Input: part model. Units: mm. Frame: model coordinates. A direction names the side the tool comes from. Give positions to 0.01 mm unless a question says otherwise; leave off trailing zeros. Write each loop counter-clockwise with the first axis right and the second up, starting at its lowest first coordinate (ties: lowest second). Pieces come first, ordered by that corner, then holes.
```python
from build123d import *

# Parameters (mm, degrees)
F0_W      = 127
F0_H      = 304.8
F0_W_2    = 76.2
F0_H_2    = 182.88
F1_DEPTH  = 19.05
F2_W      = 101.6
F2_H      = 25.4
F3_DEPTH  = 41.91
F4_W      = 101.6
F4_H      = 208.28
F5_DEPTH  = 12.7
F6_W      = 114.3
F6_H      = 35.56
F7_DEPTH  = 12.7
F8_W      = 85.55
F8_H      = 192.23
F8_W_2    = 79.2
F8_H_2    = 185.88
F8_W_3    = 88.9
F8_H_3    = 3.175
F9_DEPTH  = 3.175
F10_W     = 85.55
F10_H     = 192.23
F10_W_2   = 79.2
F10_H_2   = 185.88
F10_W_3   = 88.9
F10_H_3   = 3.175
F11_DEPTH = 3.175
F13_D     = 15.24
F14_R     = 6.35
F15_W     = 6.35
F15_H     = 242.316
F16_DEPTH = 12.7
F18_DEPTH = 25.4
F19_R     = 3.175
F20_DEPTH = 12.7
F21_R     = 3.175
F22_DEPTH = 12.7


with BuildPart() as f1:
    # F0 (on Front) → F1 (new body, symmetric)
    with BuildSketch(Plane.XZ):
        Rectangle(F0_W, F0_H)
        Rectangle(F0_W_2, F0_H_2, mode=Mode.SUBTRACT)
    extrude(amount=F1_DEPTH, both=True)

    # F2 (on face) → F3 (cut)
    with BuildSketch(Plane(origin=(0, 0, -152.4), x_dir=(1, 0, 0), z_dir=(0, 0, -1))):
        Rectangle(F2_W, F2_H)
    extrude(amount=-F3_DEPTH, mode=Mode.SUBTRACT)

    # F4 (on Front) → F5 (cut, symmetric)
    with BuildSketch(Plane.XZ):
        Rectangle(F4_W, F4_H)
    extrude(amount=F5_DEPTH, both=True, mode=Mode.SUBTRACT)

    # F6 (on Front) → F7 (cut, symmetric)
    with BuildSketch(Plane.XZ):
        with Locations((0, 128.27)):
            Rectangle(F6_W, F6_H)
    extrude(amount=F7_DEPTH, both=True, mode=Mode.SUBTRACT)

    # F8 (on face) → F9 (join)
    with BuildSketch(Plane.XZ.offset(-12.7)):
        Rectangle(F8_W, F8_H)
        Rectangle(F8_W_2, F8_H_2, mode=Mode.SUBTRACT)
        with Locations((0, -149.3139)):
            Rectangle(F8_W_3, F8_H_3)
    extrude(amount=F9_DEPTH)

    # F10 (on face) → F11 (join)
    with BuildSketch(Plane(origin=(0, -12.7, 0), x_dir=(-1, 0, 0), z_dir=(0, 1, 0))):
        Rectangle(F10_W, F10_H)
        Rectangle(F10_W_2, F10_H_2, mode=Mode.SUBTRACT)
        with Locations((0, -149.3139)):
            Rectangle(F10_W_3, F10_H_3)
    extrude(amount=F11_DEPTH)

    # F13 (through all)
    with Locations(Plane.XZ.offset(19.05)):
        with Locations((0, 128.27)):
            Hole(F13_D / 2)

    # F14
    f14_edges = [f1.edges().sort_by_distance(p)[0] for p in [
        (-57.15, 0, 146.05),
        (-57.15, 0, 110.49),
        (57.15, 0, 110.49),
        (57.15, 0, 146.05),
        (-50.8, 0, 104.14),
        (50.8, 0, 104.14),
        (-50.8, 0, -110.49),
        (-50.8, 0, -104.14),
        (50.8, 0, -110.49),
        (50.8, 0, -104.14),
        (-42.775, -11.1125, 96.115),
        (-38.1, 15.875, 91.44),
        (-38.1, -15.875, 91.44),
        (-39.6, -11.1125, 92.94),
        (38.1, 15.875, 91.44),
        (38.1, -15.875, 91.44),
        (42.775, -11.1125, 96.115),
        (39.6, -11.1125, 92.94),
        (-39.6, 11.1125, 92.94),
        (-42.775, 11.1125, 96.115),
        (42.775, 11.1125, 96.115),
        (39.6, 11.1125, 92.94),
        (38.1, 15.875, -91.44),
        (38.1, -15.875, -91.44),
        (39.6, 11.1125, -92.94),
        (42.775, 11.1125, -96.115),
        (42.775, -11.1125, -96.115),
        (39.6, -11.1125, -92.94),
        (-39.6, 11.1125, -92.94),
        (-38.1, 15.875, -91.44),
        (-38.1, -15.875, -91.44),
        (-42.775, 11.1125, -96.115),
        (-39.6, -11.1125, -92.94),
        (-42.775, -11.1125, -96.115),
        (-63.5, 0, 152.4),
        (63.5, 0, 152.4),
        (-63.5, 0, -152.4),
        (63.5, 0, -152.4),
    ]]
    fillet(f14_edges, radius=F14_R)

    # F15 (on Front) → F16 (cut)
    with BuildSketch(Plane.XZ):
        with Locations((47.625, -4.318)):
            Rectangle(F15_W, F15_H)
    extrude(amount=-F16_DEPTH, mode=Mode.SUBTRACT)

    # F17 (on face) → F18 (cut)
    with BuildSketch(Plane(origin=(0, 19.05, 0), x_dir=(-1, 0, 0), z_dir=(0, 1, 0))):
        with BuildLine():
            ThreePointArc((-19.752405, 138.177781), (-21.22344, 142.609762), (-25.655422, 141.138727))
            ThreePointArc((-25.655422, 141.138727), (-28.68965, 127.428104), (-24.856661, 113.919))
            ThreePointArc((-24.856661, 113.919), (-20.346045, 112.710384), (-19.137429, 117.221))
            ThreePointArc((-19.137429, 117.221), (-22.088492, 127.621815), (-19.752405, 138.177781))
        make_face()
    extrude(amount=-F18_DEPTH, mode=Mode.SUBTRACT)

    # F19 (on face) → F20 (cut)
    with BuildSketch(Plane.XZ.offset(19.05)):
        with Locations((21.997045, 115.57)):
            Circle(F19_R)
    extrude(amount=-F20_DEPTH, mode=Mode.SUBTRACT)

    # F21 (on Front) → F22 (cut, symmetric)
    with BuildSketch(Plane.XZ):
        with Locations((-58.42, 101.346)):
            Circle(F21_R)
        with Locations((58.42, -105.41)):
            Circle(F21_R)
    extrude(amount=F22_DEPTH, both=True, mode=Mode.SUBTRACT)


solid = f1.part
```
Item 1: Set-up query: faces 4 (the flat face through (48, 0, -107)), 5 (the flat face through (-50.8, 0, -1)), 6 (the cylindrical face through (36.29, -15.83, 89.53)). Return all of +Z, -Z, +X, -X, +Y, -Y with unobstructed straight access to the full face (end or side cutting, diameter ignored); none if empty.
Item 2: Mould query, pull axis Y, two halves, no side actions, for faces 1 (the cylindrical face through (57.73, -0.18, -108.51)), 2 (the flat face through (0, 16, 91.44)), 3 (the flat face through (41, -19.05, 2)). Classes: +Y half, -Y half, draft (parallel to the pull), parting line (faces both ways), or undercut.
Item 3: Ray query, line 1 (Z direction, x = 11, y = -7.5); line 2 (X direction, y = 16, z = 128); line 3 (Z direction, x = 29, y = -14.5). Return the intervals inside material, ascending.
Item 4: Section B-B (z = 128.27). Return loops of the section in (x, y).
Item 5: Section C-C (x = 0). Give the number of separate pieces and of enclosed holes in the cut face, and give its area (3 significant figures).
Item 6: Pin query (flat end, axial travel): pin 1 (1.6 mm diameter, centred on y = 10.5, z = -149, fed in from +X); pin 2 (20.5 mm diameter, centred on x = 10.5, y = -3, fed in from -Z); pin 3 (7.5 mm diameter, centred on x = 14, y = 0.5, fed in from -Z). Return the tip coordinate at first contact, or that it passes through.
Solved:
1. face 4: -Z
1. face 5: none
1. face 6: +Y, -Y
2. face 1: undercut
2. face 2: draft
2. face 3: -Y half
3. line 1: z = -110.49 to -104.14, 104.14 to 110.49, 146.05 to 152.4
3. line 2: x = -63.5 to -7.62, 7.62 to 22.1, 28.7 to 63.5
3. line 3: z = -152.4 to -91.44, 91.44 to 152.4
4. outline: (-63.5, -19.05) - (-7.62, -19.05) - (-7.62, -12.7) - (-57.15, -12.7) - (-57.15, 12.7) - (-7.62, 12.7) - (-7.62, 19.05) - (-63.5, 19.05) - close; (7.62, -19.05) - (63.5, -19.05) - (63.5, 19.05) - (28.7, 19.05) - (28.7, 12.7) - (57.15, 12.7) - (57.15, -12.7) - (7.62, -12.7) - close; (7.62, 12.7) - (22.1, 12.7) - (22.1, 19.05) - (7.62, 19.05) - close
5. separate pieces: 3
5. enclosed holes: 0
5. area: 1,900 mm2
6. pin 1: stops at x = 63.12
6. pin 2: stops at z = -152.4
6. pin 3: stops at z = -110.49
